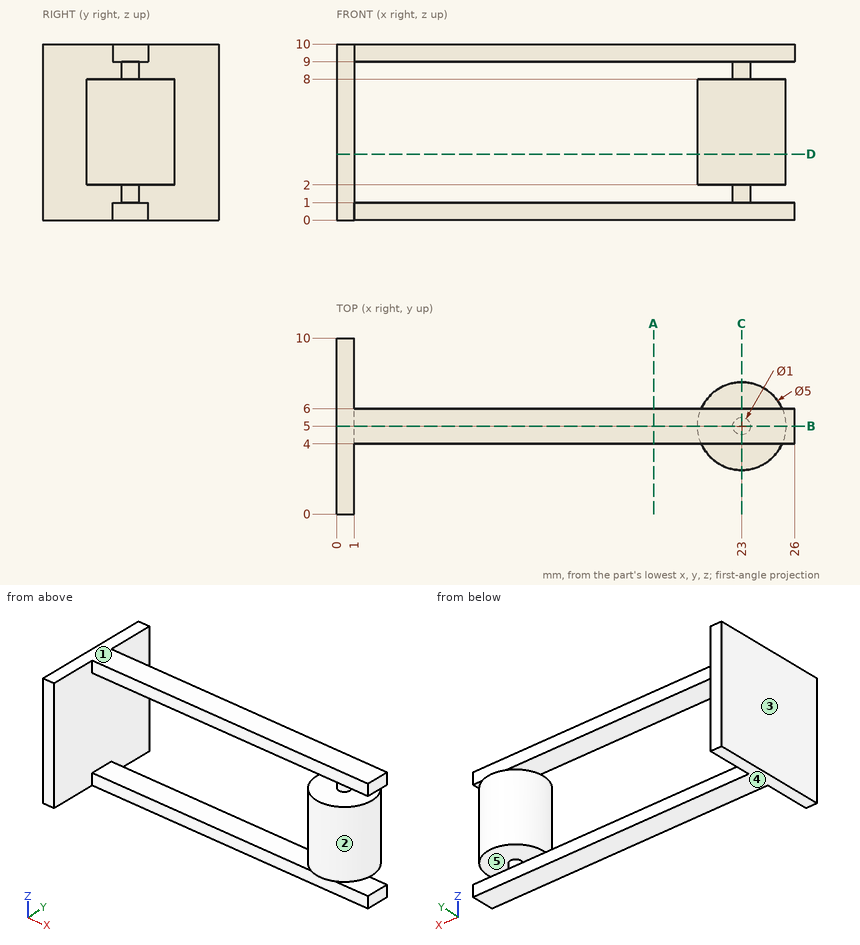
Part print with two shaded views. Sizes in mm from the minimum x, y, z corner. A direction names the side the tool comes from. Round coordinates to 2 decimals unless told otherwise and drop trailing zeros. Write each loop counter-clockwise with the first axis right and the second up, starting at its lowest first coordinate (ties: lowest second). Pieces come first, ordered by that corner, then holes. Notation, with made-up numbers: M -3.75,4.25 L 10.25,4.25 A14 cw 10.25,11.25 Z; hole C 55,11.5 d8. An arc over 180 degrees is marked long. Use CSV: the item, a comma, the result in double quotes.
1. Wall check: probe 1 along Z at (x, y) = (6, 5.25); probe 2 along X at (y, z) = (0.75, 8.75); probe 3 along X at (y, z) = (3.5, 4.5). Give the ranges that are in metal, low to high. Write a range as from..to.
Reply:
probe 1,"z = 0..1, 9..10"
probe 2,"x = 0..1"
probe 3,"x = 0..1, 21..25"
2. Saw through at C-C (x = 23). Give the cut face in (y, z).
Reply:
outline,"M 2.5,2 L 4.5,2 L 4.5,1 L 4,1 L 4,0 L 6,0 L 6,1 L 5.5,1 L 5.5,2 L 7.5,2 L 7.5,8 L 5.5,8 L 5.5,9 L 6,9 L 6,10 L 4,10 L 4,9 L 4.5,9 L 4.5,8 L 2.5,8 Z"
3. Two-plate mould, pull along Z, no slides. Class the marked faces 3, 4 and 5: +Z half, -Z half, draft (parallel to the pull), parting line (faces both ways), or undercut.
Reply:
face 3,"draft"
face 4,"-Z half"
face 5,"undercut"
4. Saw through at B-B (y = 5). Give the cut face in (x, z), plus the area to 3 significant figures.
Reply:
outline,"M 0,0 L 26,0 L 26,1 L 23.5,1 L 23.5,2 L 25.5,2 L 25.5,8 L 23.5,8 L 23.5,9 L 26,9 L 26,10 L 0,10 Z; hole M 1,1 L 22.5,1 L 22.5,2 L 20.5,2 L 20.5,8 L 22.5,8 L 22.5,9 L 1,9 Z"
area,"92.0 mm²"
5. Saw through at A-A (x = 18). Give the cut face in (y, z), plus the area to 3 significant figures.
Reply:
outline,"M 4,0 L 6,0 L 6,1 L 4,1 Z; M 4,9 L 6,9 L 6,10 L 4,10 Z"
area,"4.00 mm²"
6. Tool access for the marked faces 1 and 2: list every direction of +Z, -Z, +X, -X, +Y, -Y with a clear straight run to the whole face (end or side of a thin tool).
Reply:
face 1,"+Z, +X, -X, +Y, -Y"
face 2,"none"
7. Flat gauge pins, fed straight in: pin 1 (0.5 mm diameter, centred on x = 19, z = 0.5, fed in from -Y); pin 2 (3 mm diameter, centred on x = 14.5, z = 8, fed in from +Y); pin 3 (1.5 mm diameter, centred on x = 15, y = 7, fed in from -Z). Where does each tip first touch, or does it go through?
Reply:
pin 1,"stops at y = 4"
pin 2,"stops at y = 6"
pin 3,"passes through"
8. Saw through at D-D (z = 3.75). Give the cut face in (x, y), plus the area to 3 significant figures.
Reply:
outline,"M 0,0 L 1,0 L 1,10 L 0,10 Z; C 23,5 d5"
area,"29.6 mm²"
